Autodesk Inventor part; units mm, degrees
ref_plane "Work Plane1" through (0, -36, 0) normal (0, 1, 0) x (-1, 0, 0)
ref_plane "YZ Plane" through (0, 0, 0) normal (1, 0, 0) x (0, 1, 0)
ref_plane "XY Plane" through (0, 0, 0) normal (0, 0, 1) x (1, 0, 0)
sketch "Sketch1" plane through (0, 0, 0) normal (0, 0, 1) x (1, 0, 0)
  circle A0 centre (0, 0) radius 30
  dimension "d0" = 60
extrude "Extrusion1" add sketch "Sketch1" along normal mid plane 88
sketch "Sketch2" plane through (0, 0, 0) normal (0, 1, 0) x (-1, 0, 0)
  line L0 (51.4648, 0) -> (-98.7887, 0)
  line L1 (0, -61.6) -> (0, 61.6)
  point P0 (0, 0)
  point P1 (-48, 0)
  dimension "d11" = 48
ref_plane "Work Plane1" through (0, -36, 0) normal (0, 1, 0) x (-1, 0, 0)
sketch "Sketch3" plane through (0, -36, 0) normal (0, 1, 0) x (-1, 0, 0)
  line L0 (12, -28) -> (-60, -28)
  line L1 (-60, -28) -> (-60, 28)
  line L2 (-60, 28) -> (12, 28)
  line L3 (12, 28) -> (12, -28)
  line L4 (12, -28) -> (-60, 28) construction
  line L5 (-60, -28) -> (12, 28) construction
  line L6 (47.0012, 0) -> (-72.0071, 0)
  point P0 (0, 0)
  point P1 (-24, 0)
  point P2 (-24, 0)
  point P3 (-48, 0)
  dimension "d13" = 12
  dimension "d14" = 56
  dimension "d15" = 60
extrude "Extrusion2" add sketch "Sketch3" against normal blind 8
sketch "Sketch4" plane through (0, -36, 0) normal (0, 1, 0) x (1, 0, 0)
  line L0 (-12, -36) -> (20, -36)
  line L1 (20, -36) -> (20, 36)
  line L2 (20, 36) -> (-12, 36)
  line L3 (-12, 36) -> (-12, -36)
  line L4 (-12, -36) -> (20, 36) construction
  line L5 (20, -36) -> (-12, 36) construction
  line L6 (-48, 0) -> (78, 0)
  line L7 (-12, -28) -> (-12, 28)
  line L8 (60, -28) -> (-12, -28)
  point P0 (0, 0)
  point P1 (4, 0)
  point P2 (4, 0)
  dimension "d18" = 32
  dimension "d19" = 8
extrude "Extrusion3" add sketch "Sketch4" along normal blind 80
sketch "Sketch5" plane through (0, -44, 0) normal (0, -1, 0) x (1, 0, 0)
  line L0 (60, -28) -> (60, 28)
  line L1 (4, 20) -> (60, 20)
  line L2 (60, 20) -> (60, -20)
  line L3 (60, -20) -> (4, -20)
  line L4 (4, -20) -> (4, 20)
  line L5 (4, 20) -> (60, -20) construction
  line L6 (60, 20) -> (4, -20) construction
  line L7 (-48, 0) -> (78, 0)
  point P0 (0, 0)
  point P1 (32, 0)
  point P2 (32, 0)
  dimension "d22" = 40
  dimension "d23" = 56
extrude "Extrusion4" add sketch "Sketch5" along normal blind 96
ref_plane "Work Plane2" through (0, 184, 0) normal (0, 1, 0) x (-1, 0, 0)
ref_plane "UCS3: YZ Plane" through (0, 0, 0) normal (1, 0, 0) x (0, 1, 0)
ref_plane "UCS3: XZ Plane" through (0, 0, 0) normal (0, 1, 0) x (0, 0, 1)
ref_plane "UCS3: XY Plane" through (0, 0, 0) normal (0, 0, 1) x (1, 0, 0)
properties part number "link_3"
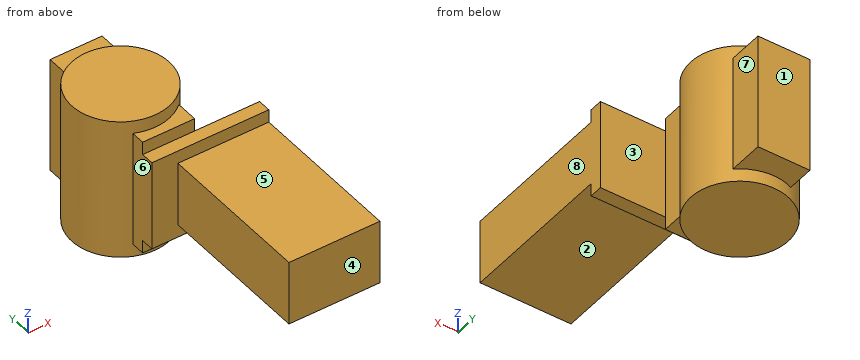
Source: CAD feature listing. Evaluate the final solid. Frame: model axes, mm. Face numbers are marked on the shaded views. A direction names the side the tool comes from. Round coordinates to 2 decimals unless told otherwise and drop trailing zeros. Loops run counter-clockwise (first coordinate to the right, second up) from the corner with the lowest first, then second, coordinate; pieces in that order, holes last.
Q1. Section C-C, the plane y = 0. Return loops of the section in (x, z), plus the area to 3 significant figures.
Q2. First-contact query: P1, Ø12, axis at y = -97.5, z = 8.5, coming from the -X side; P2, Ø5, axis at y = 34.5, z = 8, coming from the -X side; P3, Ø4, axis at x = 4.5, z = 31.5, coming from the -Y side; P4, Ø8, axis at y = -81.5, z = 27, coming from the -X side. Flat tips, straight axial feed; report the tip coordinate or a pass-through.
Q3. Section B-B, the plane x = 0. Return loops of the section in (y, z).
Q4. Mould query, pull axis Y, two halves, no side actions, for the marked faces 1, 2, 3 and 4. Classes: pulls with the +Y half, pulls with the -Y half, needs draft (parallel to the pull), parting line crosses it, or undercut.
Q5. Ray query, line 1 (Y direction, x = -1.5, z = 25); line 2 (Y direction, x = 34, z = 14); line 3 (X direction, y = -41.5, z = 16.5). Return the intervals inside material, ascending.
Q6. Access query for the marked faces 5, 6, 7 and 8. Directions: +Z, -Z, +X, -X, +Y, -Y. A direction counts if a zero-diameter tool reaches every point of the face in a straight line with its end or side. Return the directions, or none.
Q7. Section A-A, the plane z = 32.5. Return loops of the section in (x, y).
Q8. Section D-D, the plane z = -13. Return loops of the section in (x, y), plus the area to 3 significant figures.
Solutions:
1. outline: (-30, -44) - (30, -44) - (30, 44) - (-30, 44) - close
1. area: 5,280 mm2
2. P1: stops at x = 4
2. P2: stops at x = -12
2. P3: stops at y = -36
2. P4: passes through
3. outline: (-44, -28) - (-36, -28) - (-36, -36) - (-30, -36) - (-30, -44) - (30, -44) - (30, -36) - (44, -36) - (44, 36) - (30, 36) - (30, 44) - (-30, 44) - (-30, 36) - (-36, 36) - (-36, 28) - (-44, 28) - close
4. face 1: pulls with the +Y half
4. face 2: needs draft
4. face 3: undercut
4. face 4: pulls with the -Y half
5. line 1: y = -44 to 44
5. line 2: y = -140 to -36
5. line 3: x = -12 to 60
6. face 5: +Z, +X, -X, -Y
6. face 6: +Z, -Z, -X, -Y
6. face 7: +Z, -Z, +X, +Y
6. face 8: +Z, -Z, +X, +Y, -Y
7. outline: (-12, -36) - (20, -36) - (20, -22.36) arc R30 ccw to (20, 22.36) - (20, 44) - (-12, 44) - (-12, 27.5) arc R30 ccw to (-12, -27.5) - close
8. outline: (-12, -44) - (4, -44) - (4, -140) - (60, -140) - (60, -36) - (20, -36) - (20, -22.36) arc R30 ccw to (20, 22.36) - (20, 44) - (-12, 44) - (-12, 27.5) arc R30 ccw to (-12, -27.5) - close
8. area: 9,540 mm2
